Here's how the part is built. I have some questions about the finished solid (model axes, mm). Round coordinates to 2 decimals unless told otherwise and drop trailing zeros. Order: outer loops, then holes, each group sorted by start corner. A loop starts at its lowest first (then second) coordinate and runs counter-clockwise, first axis right, second up. Notation, with made-up numbers: M 44,75.5 L 57,75.5 A25 ccw 57,90.5 Z; hole C 30.25,-14 d4. An arc over 180 degrees is marked long. Use one line per item in the form item = value. Start each with the question number.
```python
from build123d import *

# Parameters (mm, degrees)
SKETCH_2_R      = 5
EXTRUDE_1_DEPTH = 10


with BuildPart() as part:
    # 草图2 → 凸台-拉伸1 (new body)
    with BuildSketch(Plane.XY):
        with BuildLine():
            Line((0, 10), (200, 10))
            ThreePointArc((200, 10), (210, 0), (200, -10))
            Line((200, -10), (0, -10))
            ThreePointArc((0, -10), (-10, 0), (0, 10))
        make_face()
        Circle(SKETCH_2_R, mode=Mode.SUBTRACT)
        with Locations((200, 0)):
            Circle(SKETCH_2_R, mode=Mode.SUBTRACT)
        with Locations((100, 0)):
            Circle(SKETCH_2_R, mode=Mode.SUBTRACT)
    extrude(amount=EXTRUDE_1_DEPTH)


solid = part.part
```
1) If we section it at A-A on y = 0: Write out the boundary of the cut face in (x, z).
2) If we section it at C-C on z = 8.25: Write out the boundary of the cut face in (x, y).
3) Will these pins go through, and if not, where does the flat tip stop? pin 1 Ø6 at (y, z) = (5, 3.5) entering from +X; pin 2 Ø1 at (y, z) = (5, 2.5) entering from +X.
4) If I drill on line 1 (X direction, y = 0.5, z = 8.5); line 2 (Y direction, x = 100, z = 3.5); line 3 (X direction, y = 4.5, z = 0.5), over which ranges is the centre line in solid material (lowest first)?
5) If we mould it in two halves opening along Y, with no side actions, what happens to faces 1 (the cylindrical face through (-1.08, -4.88, 4.93)), 2 (the flat face through (102, 7, 10)), 3 (the cylindrical face through (204.77, 1.5, 4.93)), 4 (the cylindrical face through (-10, 0, 5))? For each: +Y half, -Y half, draft (parallel to the pull), parting line (faces both ways), or undercut.
6) If we section it at B-B on x = 100: Write out the boundary of the cut face in (y, z).
Completed:
q1.outline = M -10,0 L -5,0 L -5,10 L -10,10 Z; M 5,0 L 95,0 L 95,10 L 5,10 Z; M 105,0 L 195,0 L 195,10 L 105,10 Z; M 205,0 L 210,0 L 210,10 L 205,10 Z
q2.outline = M 0,-10 L 200,-10 A10 ccw 200,10 L 0,10 A10 ccw Z; hole C 0,0 d10; hole C 100,0 d10; hole C 200,0 d10
q3.pin_1 = 209.8
q3.pin_2 = 208.93
q4.line_1 = -9.99 to -4.97, 4.97 to 95.03, 104.97 to 195.03, 204.97 to 209.99
q4.line_2 = -10 to -5, 5 to 10
q4.line_3 = -8.93 to -2.18, 2.18 to 97.82, 102.18 to 197.82, 202.18 to 208.93
q5.face_1 = undercut
q5.face_2 = draft
q5.face_3 = undercut
q5.face_4 = parting line
q6.outline = M -10,0 L -5,0 L -5,10 L -10,10 Z; M 5,0 L 10,0 L 10,10 L 5,10 Z
